Geometry check sheet. Reference: the model listing, model coordinates, mm. Give positions to 0.01 mm unless a question says otherwise; leave off trailing zeros. Loops run counter-clockwise (first coordinate to the right, second up) from the corner with the lowest first, then second, coordinate; pieces in that order, holes last. Notation, with made-up numbers: (56.25, -4) - (114.25, -4) arc R26 cw to (114.25, 14) - close; hole circle Ø6 at (-28, -6.5). An arc over 180 degrees is marked (long way). Use a Markdown table: item, result. Add a question column.
1. Cross-section at C-C on y = 39. Enter the section's corners in (x, z), and give its area (3 significant figures).
2. Cross-section at D-D on z = 62. Enter the section's corners in (x, y).
3. Material ranges on L1, parallel to Z at x = 1.2, y = 43; L2, parallel to Z at x = 0.4, y = 95; L3, parallel to Y at x = 1.95, z = 26, recorded low to high.
4. Cross-section at B-B on x = 1.1. Enter the section's corners in (y, z), and give its area (3 significant figures).
5. Cross-section at A-A on y = 133.5. Enter the section's corners in (x, z), and give its area (3 significant figures).
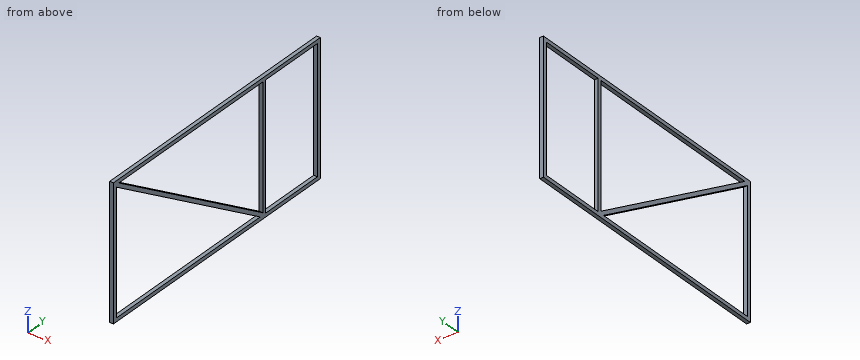
from build123d import *

# Parameters (mm, degrees)
F0_W     = 144
F0_H     = 72
F0_W_2   = 36
F0_H_2   = 68
F1_DEPTH = 2


with BuildPart() as f1:
    # F0 (on Right) → F1 (new body)
    with BuildSketch(Plane.YZ):
        with Locations((72, 36)):
            Rectangle(F0_W, F0_H)
        Polygon((2, 2), (2, 68.79815), (102.197224, 2), align=None, mode=Mode.SUBTRACT)
        Polygon((104, 70), (104, 3.20185), (3.802776, 70), align=None, mode=Mode.SUBTRACT)
        with Locations((124, 36)):
            Rectangle(F0_W_2, F0_H_2, mode=Mode.SUBTRACT)
    extrude(amount=F1_DEPTH)


solid = f1.part
Values found:
| question | item | result |
|---|---|---|
| 1 | outline | (0, 0) - (2, 0) - (2, 2) - (0, 2) - close; (0, 44.13) - (2, 44.13) - (2, 46.54) - (0, 46.54) - close; (0, 70) - (2, 70) - (2, 72) - (0, 72) - close |
| 1 | area | 12.8 mm2 |
| 2 | outline | (0, 0) - (2, 0) - (2, 2) - (0, 2) - close; (0, 12.2) - (2, 12.2) - (2, 15.8) - (0, 15.8) - close; (0, 104) - (2, 104) - (2, 106) - (0, 106) - close; (0, 142) - (2, 142) - (2, 144) - (0, 144) - close |
| 3 | L1 | z = 0 to 2, 41.46 to 43.87, 70 to 72 |
| 3 | L2 | z = 0 to 2, 6.8 to 9.2, 70 to 72 |
| 3 | L3 | y = 0 to 2, 66.2 to 69.8, 104 to 106, 142 to 144 |
| 4 | outline | (0, 0) - (144, 0) - (144, 72) - (0, 72) - close; hole (2, 2) - (102.2, 2) - (2, 68.8) - close; hole (3.8, 70) - (104, 3.2) - (104, 70) - close; hole (106, 2) - (142, 2) - (142, 70) - (106, 70) - close |
| 4 | area | 1,230 mm2 |
| 5 | outline | (0, 0) - (2, 0) - (2, 2) - (0, 2) - close; (0, 70) - (2, 70) - (2, 72) - (0, 72) - close |
| 5 | area | 8.00 mm2 |
